Can you work these out from the model? Positions are in its coordinate system, mm. Face numbers are marked on the shaded views. A direction names the side the tool comes from. Round coordinates to 2 decimals unless told otherwise and drop trailing zeros. Loops run counter-clockwise (first coordinate to the right, second up) from the corner with the lowest first, then second, coordinate; pieces in that order, holes last.
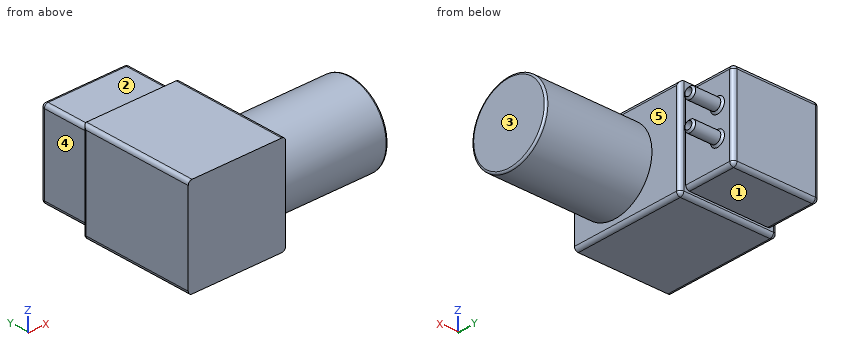
```python
from build123d import *

# Parameters (mm, degrees)
ESQUISSE1_W        = 51
ESQUISSE1_H        = 51
BOSS_EXTRU_1_DEPTH = 60
ESQUISSE2_W        = 45
ESQUISSE2_H        = 45
BOSS_EXTRU_2_DEPTH = 27
ESQUISSE3_R        = 21.05
BOSS_EXTRU_3_DEPTH = 55.5
ESQUISSE4_R        = 4
BOSS_EXTRU_4_DEPTH = 1
ESQUISSE5_R        = 3
ESQUISSE5_R_2      = 2
BOSS_EXTRU_5_DEPTH = 14.2
CHANFREIN1_SIZE    = 1
CONG_1_R           = 2
CONG_2_R           = 2
CONG_3_R           = 1


with BuildPart() as part:
    # Esquisse1 → Boss.-Extru.1 (new body)
    with BuildSketch(Plane(origin=(0, 0, 0), x_dir=(1, 0, 0), z_dir=(0, 1, 0))):
        with Locations((25.5, 25.5)):
            Rectangle(ESQUISSE1_W, ESQUISSE1_H)
    extrude(amount=BOSS_EXTRU_1_DEPTH)

    # Esquisse2 → Boss.-Extru.2 (add)
    with BuildSketch(Plane(origin=(0, 60, 0), x_dir=(1, 0, 0), z_dir=(0, 1, 0))):
        with Locations((25.5, 25.5)):
            Rectangle(ESQUISSE2_W, ESQUISSE2_H)
    extrude(amount=BOSS_EXTRU_2_DEPTH)

    # Esquisse3 → Boss.-Extru.3 (add)
    with BuildSketch(Plane(origin=(51, 0, 0), x_dir=(0, 0, -1), z_dir=(1, 0, 0))):
        with Locations(Location((25.5, 23, 0), (0, 0, 180))):
            Circle(ESQUISSE3_R)
    extrude(amount=BOSS_EXTRU_3_DEPTH)

    # Esquisse4 → Boss.-Extru.4 (add)
    with BuildSketch(Plane(origin=(48, 0, 0), x_dir=(0, 0, -1), z_dir=(1, 0, 0))):
        with Locations(Location((18.1, 78, 0), (0, 0, 180))):
            Circle(ESQUISSE4_R)
        with Locations(Location((32.9, 78, 0), (0, 0, 180))):
            Circle(ESQUISSE4_R)
    extrude(amount=BOSS_EXTRU_4_DEPTH)

    # Esquisse5 → Boss.-Extru.5 (add)
    # profile 1 of 2: a face of its own
    with BuildSketch(Plane(origin=(49, 0, 0), x_dir=(0, 0, -1), z_dir=(1, 0, 0))):
        with Locations((18.1, 78)):
            Circle(ESQUISSE5_R)
        with Locations((18.1, 78)):
            Circle(ESQUISSE5_R_2, mode=Mode.SUBTRACT)
    # profile 2 of 2: a face of its own
    with BuildSketch(Plane(origin=(49, 0, 0), x_dir=(0, 0, -1), z_dir=(1, 0, 0))):
        with Locations((32.9, 78)):
            Circle(ESQUISSE5_R)
        with Locations((32.9, 78)):
            Circle(ESQUISSE5_R_2, mode=Mode.SUBTRACT)
    extrude(amount=BOSS_EXTRU_5_DEPTH)

    # Chanfrein1
    chanfrein1_edges = [part.edges().sort_by_distance(p)[0] for p in [
        (49, 78, -22.1),
        (49, 78, -36.9),
        (63.2, 78, -15.1),
        (63.2, 78, -29.9),
    ]]
    chamfer(chanfrein1_edges, length=CHANFREIN1_SIZE - 0.0001)  # a hair under: the kernel refuses the full size

    # Congé1
    cong_1_edges = [part.edges().sort_by_distance(p)[0] for p in [
        (3, 73.5, -48),
        (3, 73.5, -3),
        (48, 73.5, -3),
        (48, 73.5, -48),
        (3, 87, -25.5),
        (25.5, 87, -3),
        (48, 87, -25.5),
        (25.5, 87, -48),
    ]]
    fillet(cong_1_edges, radius=CONG_1_R)

    # Congé2
    cong_2_edges = [part.edges().sort_by_distance(p)[0] for p in [
        (51, 60, -25.5),
        (25.5, 60, -51),
        (0, 60, -25.5),
        (0, 30, -51),
        (51, 30, -51),
        (51, 30, 0),
        (0, 30, 0),
    ]]
    fillet(cong_2_edges, radius=CONG_2_R)

    # Congé3
    cong_3_edges = [part.edges().sort_by_distance(p)[0] for p in [
        (106.5, 23, -46.55),
    ]]
    fillet(cong_3_edges, radius=CONG_3_R)


solid = part.part
```
(1) Suppose I cut it at A-A (x = 33). Write out the boundary of the cut face in (y, z), then the cut area to 3 significant figures.
(2) Suppose I cut it at C-C (y = 52). Write out the boundary of the cut face in (x, z), then the cut area to 3 significant figures.
(3) If I drill on line 1 (Y direction, x = 52.75, z = -18.1); line 2 (Y direction, x = 53, z = -32); line 3 (X direction, y = 43, z = -11), over which ranges is the centre line in solid material (lowest first)?
(4) Suppose I cut it at D-D (y = 70.5). Write out the boundary of the cut face in (x, z).
(5) Suppose I cut it at B-B (y = 23). Write out the boundary of the cut face in (x, z), then the cut area to 3 significant figures.
(6) For pin 1 (4.5 mm diameter, centred on y = 77, z = -32.5, fed in from +X); pin 2 (7.5 mm diameter, centred on y = 71.5, z = -27, fed in from +X); pin 3 (8 mm diameter, centred on x = 62, z = -29.5, fed in from +Y), each with a flat end and sliding along its axis, tell me the tip position at first contact or that it passes through.
(7) Which directions (+Z, -Z, +X, -X, +Y, -Y) give clear straight access to the entire face, cutting with the end or side of a thin tool? Please do the marked faces 1, 2, 3, 4 and 5.
Check result:
1. outline: (0, -51) - (58, -51) arc R2 ccw to (60, -49) - (60, -48) - (85, -48) arc R2 ccw to (87, -46) - (87, -5) arc R2 ccw to (85, -3) - (60, -3) - (60, 0) - (0, 0) - close
1. area: 4,270 mm2
2. outline: (0, -49) arc R2 ccw to (2, -51) - (49, -51) arc R2 ccw to (51, -49) - (51, -2) arc R2 ccw to (49, 0) - (2, 0) arc R2 ccw to (0, -2) - close
2. area: 2,600 mm2
3. line 1: y = 3.29 to 42.71, 75 to 76, 80 to 81
3. line 2: y = 2.98 to 43.02, 75.14 to 76.21, 79.79 to 80.86
3. line 3: x = 0 to 51
4. outline: (3, -46) arc R2 ccw to (5, -48) - (46, -48) arc R2 ccw to (48, -46) - (48, -5) arc R2 ccw to (46, -3) - (5, -3) arc R2 ccw to (3, -5) - close
5. outline: (0, -49) arc R2 ccw to (2, -51) - (49, -51) arc R2 ccw to (51, -49) - (51, -46.55) - (105.5, -46.55) arc R1 ccw to (106.5, -45.55) - (106.5, -5.45) arc R1 ccw to (105.5, -4.45) - (51, -4.45) - (51, -2) arc R2 ccw to (49, 0) - (2, 0) arc R2 ccw to (0, -2) - close
5. area: 4,930 mm2
6. pin 1: stops at x = 63.2
6. pin 2: stops at x = 48
6. pin 3: stops at y = 81
7. face 1: -Z, +X, -X, +Y
7. face 2: +Z, +X, -X, +Y
7. face 3: +Z, -Z, +X, +Y, -Y
7. face 4: +Z, -Z, -X, +Y
7. face 5: +X
